from build123d import *

# Parameters (mm, degrees)
F0_W           = 56.5020628273
F0_H           = 64.7920891643
F1_DEPTH       = 25.4
F3_D           = 6.35
F3_CBORE_D     = 12.7
F3_CBORE_DEPTH = 6.35
F4_T           = -2.54


with BuildPart() as f1:
    # F0 (on Top) → F1 (new body)
    with BuildSketch(Plane.XY):
        with Locations((28.2510314137, 32.3960445821)):
            Rectangle(F0_W, F0_H)
    extrude(amount=F1_DEPTH)

    # F3 (through all)
    with Locations(Plane.XY.offset(25.4)):
        with Locations((13.101497665, 18.814554438)):
            CounterBoreHole(F3_D / 2, F3_CBORE_D / 2, F3_CBORE_DEPTH)

    # F4
    f4_openings = [f1.faces().sort_by_distance(p)[0] for p in [
        (56.502063, 32.396045, 12.7),
    ]]
    offset(amount=F4_T, openings=f4_openings, kind=Kind.INTERSECTION)


solid = f1.part
Check sheet for the modelled part. Datum: model origin and axes. Units: mm. A direction names the side the tool comes from. Give positions to 0.01 mm unless a question says otherwise; leave off trailing zeros. Loops run counter-clockwise (first coordinate to the right, second up) from the corner with the lowest first, then second, coordinate; pieces in that order, holes last. Notation, with made-up numbers: M 14.5,78.5 L 52.5,78.5 A8 cw 52.5,84.5 Z; hole C 56.5,25 d9. An arc over 180 degrees is marked long. Use a Markdown table: item, result. Add a question column.
Q1. Mould release check, pull along Y, two halves, no side actions. Record for faces 4 (the cylindrical face through (6.047, 13.405, 19.729)), 5 (the flat face through (28, 0, 13)), 6 (the flat face through (0, 32, 13)): pulls with the +Y half, pulls with the -Y half, needs draft (parallel to the pull), parting line crosses it, or undercut.
Q2. Sectioned sample at A-A, the plane z = 12.25. Give the number of separate pieces and of enclosed holes in the cut face, then the cut area to 3 significant figures.
Q3. Go/stop test with flat-tipped pins: pin 1 (2 mm diameter, centred on x = 32, y = 16, fed in from -Z); pin 2 (1.5 mm diameter, centred on y = 37, z = 7, fed in from +X); pin 3 (5 mm diameter, centred on y = 24, z = 11.5, fed in from +X). Record where each tip stops, or that it passes through.
Q4. Tool access check on faces 1 (the flat face through (29, 2.54, 13)), 2 (the flat face through (10, 17, 19.05)), 3 (the cylindrical face through (14.34, 13.235, 9.427)). Record the directions out of +Z, -Z, +X, -X, +Y, -Y that give a thin tool (end or side, any length) a straight path to the whole face; none if there is none.
Q5. Sectioned sample at B-B, the plane x = 52. Record the cut outline in (y, z), then the cut area to 3 significant figures.
Q6. Scan lines: line 1 along Z through (x, y) = (40, 34.5); line 2 along Y through (x, z) = (3.5, 10); line 3 along Y through (x, z) = (11, 7.5). Record each from-to range of solid material in increasing order. Write a range as [from, to].
Q7. Sectioned sample at D-D, the plane x = 18. Record the cut outline in (y, z).
Q8. Sectioned sample at C-C, the plane y = 44.5. Record the cut outline in (x, z).
Verdict:
| question | item | result |
|---|---|---|
| 1 | face 4 | undercut |
| 1 | face 5 | pulls with the -Y half |
| 1 | face 6 | needs draft |
| 2 | separate pieces | 2 |
| 2 | enclosed holes | 1 |
| 2 | area | 510 mm^2 |
| 3 | pin 1 | z = 0 |
| 3 | pin 2 | x = 2.54 |
| 3 | pin 3 | x = 18.15 |
| 4 | face 1 | +X |
| 4 | face 2 | +Z |
| 4 | face 3 | none |
| 5 | outline | M 0,0 L 64.79,0 L 64.79,25.4 L 0,25.4 Z; hole M 2.54,2.54 L 62.25,2.54 L 62.25,22.86 L 2.54,22.86 Z |
| 5 | area | 432 mm^2 |
| 6 | line 1 | [0, 2.54], [22.86, 25.4] |
| 6 | line 2 | [0, 2.54], [62.25, 64.79] |
| 6 | line 3 | [0, 2.54], [13.5, 16.43], [21.19, 24.13], [62.25, 64.79] |
| 7 | outline | M 0,0 L 64.79,0 L 64.79,25.4 L 22.86,25.4 L 22.86,19.05 L 14.77,19.05 L 14.77,25.4 L 0,25.4 Z; hole M 2.54,2.54 L 15.87,2.54 L 15.87,16.51 L 11.4,16.51 L 11.4,22.86 L 2.54,22.86 Z; hole M 21.76,2.54 L 62.25,2.54 L 62.25,22.86 L 26.23,22.86 L 26.23,16.51 L 21.76,16.51 Z |
| 8 | outline | M 0,0 L 56.5,0 L 56.5,2.54 L 2.54,2.54 L 2.54,22.86 L 56.5,22.86 L 56.5,25.4 L 0,25.4 Z |
